Autodesk Inventor part; units mm, degrees
ref_plane "YZ Plane" through (0, 0, 0) normal (1, 0, 0) x (0, 1, 0)
ref_plane "XZ Plane" through (0, 0, 0) normal (0, 1, 0) x (-1, 0, 0)
ref_plane "XY Plane" through (0, 0, 0) normal (0, 0, 1) x (1, 0, 0)
sketch "Sketch1" plane through (0, 0, 0) normal (0, 1, 0) x (-1, 0, 0)
  circle A0 centre (0, 0) radius 1.75
  circle A1 centre (0, 0) radius 2.75
  dimension "d0" = 3.5
  dimension "d1" = 5.5
extrude "Extrusion1" add sketch "Sketch1" along normal blind 4
sketch "Sketch2" plane through (0, 4, 0) normal (0, 1, 0) x (1, 0, 0)
  circle A0 centre (0, 0) radius 1.75
  circle A1 centre (0, 0) radius 2.75
  circle A2 centre (0, 0) radius 2.75
  circle A3 centre (0, 0) radius 1.75
  circle A4 centre (0, 0) radius 2.75
  circle A5 centre (0, 0) radius 1.75
  circle A6 centre (0, 0) radius 2.75
  line L0 (-2.75, 0) -> (0, 0)
  line L1 (0, 0) -> (2.75, 0)
  arc A7 (1.75, 0) -> (-1.75, 0) centre (0, 0) ccw
  arc A8 (2.75, 0) -> (-2.75, 0) centre (0, 0) ccw
extrude "Extrusion2" add sketch "Sketch2" along normal blind 11 contours A0 L0 A1 L1 picked at (-2.3731, 0.359)
properties part number "espaciador2"
Design review of the part built by this model. Coordinates are the model's own, in mm. A direction names the side the tool comes from. Round coordinates to 2 decimals unless told otherwise and drop trailing zeros. Write each loop counter-clockwise with the first axis right and the second up, starting at its lowest first coordinate (ties: lowest second). Pieces come first, ordered by that corner, then holes. Notation, with made-up numbers: (40.5, -10) -> (85.5, -10) arc R11 ccw to (85.5, 2) -> close; hole circle Ø11 at (61, 51). An arc over 180 degrees is marked (long way). Write item = value, one per line. Start each with the question number.
1) Take a section at B-B, the plane z = -1.25. State the section outline as (x, y) points, plus the area to 3 significant figures.
2) Wall thickness on probe 1 along Z at (x, y) = (0, 5.75); probe 2 along Y at (x, z) = (-1.5, 1.6); probe 3 along X at (y, z) = (5.5, -0.6): over which ranges is each line inside the solid? List them lowest first. Write a range as from..to.
3) Mouldability with a two-part tool opening along X and no side actions: class faces 3 (the face through (2, 9, 0)), 4 (the face through (0.358, 5.728, -2.727)), 5 (the face through (0.228, 5.728, -1.735)) as +X half, -X half, draft (parallel to the pull), parting line (faces both ways), or undercut.
4) Tool access review of faces 1 (the face through (-2, 0, 0)), 2 (the face through (0, 4, 2)): name each direction out of +Z, -Z, +X, -X, +Y, -Y from which nothing blocks a thin tool from reaching the whole face with its end or side.
5) Take a section at D-D, the plane x = -2.3. State the section outline as (y, z) points, plus the area to 3 significant figures.
6) Take a section at C-C, the plane y = 10.25. State the section outline as (x, z) points.
7) Take a section at A-A, the plane x = 0. State the section outline as (y, z) points.
8) Clearance check with flat-ended pins moving along their axes: pin 1 (3 mm diameter, centred on x = 0, z = 0, fed in from +Y); pin 2 (3 mm diameter, centred on x = -2, y = 10.5, fed in from -Z); pin 3 (2 mm diameter, centred on x = 1.5, z = 1, fed in from +Y); pin 4 (1 mm diameter, centred on y = 9.5, z = -2, fed in from +X). State where each tip first meets the part, or that it passes through.
Results list:
q1.outline = (-2.45, 0) -> (-1.22, 0) -> (-1.22, 15) -> (-2.45, 15) -> close; (1.22, 0) -> (2.45, 0) -> (2.45, 15) -> (1.22, 15) -> close
q1.area = 36.7 mm²
q2.probe_1 = -2.75..-1.75
q2.probe_2 = 0..4
q2.probe_3 = -2.68..-1.64, 1.64..2.68
q3.face_3 = draft
q3.face_4 = parting line
q3.face_5 = undercut
q4.face_1 = +Z, -Z, +X, -X, -Y
q4.face_2 = +Z, +X, -X, +Y
q5.outline = (0, -1.51) -> (15, -1.51) -> (15, 0) -> (4, 0) -> (4, 1.51) -> (0, 1.51) -> close
q5.area = 28.6 mm²
q6.outline = (-2.75, 0) arc R2.75 ccw to (2.75, 0) -> (1.75, 0) arc R1.75 cw to (-1.75, 0) -> close
q7.outline = (0, -2.75) -> (15, -2.75) -> (15, -1.75) -> (0, -1.75) -> close; (0, 1.75) -> (4, 1.75) -> (4, 2.75) -> (0, 2.75) -> close
q8.pin_1 = through
q8.pin_2 = -2.7
q8.pin_3 = 4
q8.pin_4 = 2.3
